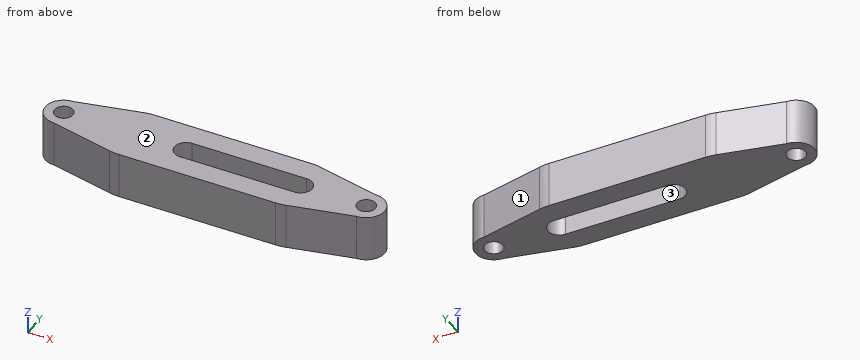
from build123d import *

# Parameters (mm, degrees)
CROQUIS1_R              = 2
SALIENTE_EXTRUIR1_DEPTH = 10
REDONDEO2_R             = 10
CORTAR_EXTRUIR1_DEPTH   = 10


with BuildPart() as part:
    # Croquis1 → Saliente-Extruir1 (new body)
    with BuildSketch(Plane.XY):
        with BuildLine():
            Line((14.815, 7.35), (51.185, 7.35))
            Line((51.185, 7.35), (66, 4))
            ThreePointArc((66, 4), (70, 0), (66, -4))
            Line((66, -4), (51.185, -7.35))
            Line((51.185, -7.35), (14.815, -7.35))
            Line((14.815, -7.35), (0, -4))
            ThreePointArc((0, -4), (-4, 0), (0, 4))
            Line((0, 4), (14.815, 7.35))
        make_face()
        Circle(CROQUIS1_R, mode=Mode.SUBTRACT)
        with Locations((66, 0)):
            Circle(CROQUIS1_R, mode=Mode.SUBTRACT)
    extrude(amount=SALIENTE_EXTRUIR1_DEPTH)

    # Redondeo2
    redondeo2_edges = [part.edges().sort_by_distance(p)[0] for p in [
        (14.815, 7.35, 5),
        (51.185, 7.35, 5),
        (51.185, -7.35, 5),
        (14.815, -7.35, 5),
    ]]
    fillet(redondeo2_edges, radius=REDONDEO2_R)

    # Croquis2 → Cortar-Extruir1 (cut)
    with BuildSketch(Plane.XY):
        with BuildLine():
            Line((51.69, 2.5), (26.69, 2.5))
            ThreePointArc((26.69, 2.5), (24.19, 0), (26.69, -2.5))
            Line((26.69, -2.5), (51.69, -2.5))
            ThreePointArc((51.69, -2.5), (54.19, 0), (51.69, 2.5))
        make_face()
    extrude(amount=CORTAR_EXTRUIR1_DEPTH, mode=Mode.SUBTRACT)


solid = part.part
Build history of the part. All positions in model axes, mm. Face numbers are marked on the shaded views. Give positions to 0.01 mm unless a question says otherwise; leave off trailing zeros. Loops run counter-clockwise (first coordinate to the right, second up) from the corner with the lowest first, then second, coordinate; pieces in that order, holes last. Notation, with made-up numbers: (-1, -4.5) - (35, -4.5) arc R20 ccw to (35, 12.5) - close; hole circle Ø7 at (-7, 13.25). An arc over 180 degrees is marked (long way). Write item = value, one per line. Start each with the question number.
1) Band-saw the part on B-B on z = 5. Give the cut face in (x, y).
2) Band-saw the part on C-C on x = 58. Give the cut face in (y, z), plus the area to 3 significant figures.
3) Pull direction X, two halves, no side cores. Call the marked faces 1, 2 and 3: +X half, -X half, draft (parallel to the pull), parting line (faces both ways), or undercut.
4) Band-saw the part on D-D on y = 5. Give the cut face in (x, z), plus the area to 3 significant figures.
5) Band-saw the part on A-A on x = 45.5. Give the cut face in (y, z).
6) Drop a flat-ended pin along its axis: pin 1 Ø6 at (y, z) = (5.5, 7.5) entering from +X. Give the stop position or say it passes through.
7) Probe probe 1 along Y at (x, z) = (48, 8.75); probe 2 along Y at (x, z) = (0, 5.75); probe 3 along X at (y, z) = (-1.5, 5.25). List the from-to ranges inside material, lowest first. Write a range as from..to.
Final values:
q1.outline = (0, -4) - (13.73, -7.1) arc R10 ccw to (15.93, -7.35) - (50.07, -7.35) arc R10 ccw to (52.27, -7.1) - (66, -4) arc R4 ccw to (66, 4) - (52.27, 7.1) arc R10 ccw to (50.07, 7.35) - (15.93, 7.35) arc R10 ccw to (13.73, 7.1) - (0, 4) arc R4 ccw to start; hole circle Ø4 at (0, 0); hole (26.69, -2.5) - (51.69, -2.5) arc R2.5 ccw to (51.69, 2.5) - (26.69, 2.5) arc R2.5 ccw to start; hole circle Ø4 at (66, 0)
q2.outline = (-5.81, 0) - (5.81, 0) - (5.81, 10) - (-5.81, 10) - close
q2.area = 116 mm²
q3.face_1 = +X half
q3.face_2 = draft
q3.face_3 = undercut
q4.outline = (4.42, 0) - (61.58, 0) - (61.58, 10) - (4.42, 10) - close
q4.area = 572 mm²
q5.outline = (-7.35, 0) - (-2.5, 0) - (-2.5, 10) - (-7.35, 10) - close; (2.5, 0) - (7.35, 0) - (7.35, 10) - (2.5, 10) - close
q6.pin_1 = 69.12
q7.probe_1 = -7.35..-2.5, 2.5..7.35
q7.probe_2 = -4..-2, 2..4
q7.probe_3 = -3.71..-1.32, 1.32..24.69, 53.69..64.68, 67.32..69.71
